```python
from build123d import *

# Parameters (mm, degrees)
EXTRUDE_1_DEPTH     = 50
SKETCH_2_R          = 13
SKETCH_2_R_2        = 2.1
CUT_EXTRUDE_1_DEPTH = 50
FILLET_1_R          = 2
SKETCH_4_R          = 12.5
SKETCH_4_R_2        = 2.5
CUT_EXTRUDE_2_DEPTH = 50
EXTRUDE_2_DEPTH     = 2
EXTRUDE_START       = -50
EXTRUDE_3_DEPTH     = 2


with BuildPart() as part:
    # 草图1 → 凸台-拉伸1 (new body)
    with BuildSketch(Plane.XY):
        with BuildLine():
            Line((0, 0), (46, 0))
            ThreePointArc((46, 0), (48.828427125, 1.171572875), (50, 4))
            Line((50, 4), (50, 50))
            Line((50, 50), (48, 50))
            Line((48, 50), (48, 4))
            ThreePointArc((48, 4), (47.414213562, 2.585786438), (46, 2))
            Line((46, 2), (0, 2))
            Line((0, 2), (0, 0))
        make_face()
    extrude(amount=EXTRUDE_1_DEPTH)

    # 草图2 → 切除-拉伸1 (cut)
    with BuildSketch(Plane(origin=(50, 0, 0), x_dir=(0, 0, -1), z_dir=(1, 0, 0))):
        with Locations((-25, 28)):
            Circle(SKETCH_2_R)
        with Locations((-25, 45.5)):
            Circle(SKETCH_2_R_2)
        with Locations((-7.5, 28)):
            Circle(SKETCH_2_R_2)
        with Locations((-25, 10.5)):
            Circle(SKETCH_2_R_2)
        with Locations((-42.5, 28)):
            Circle(SKETCH_2_R_2)
    extrude(amount=-CUT_EXTRUDE_1_DEPTH, mode=Mode.SUBTRACT)

    # 圆角1
    fillet_1_edges = [part.edges().sort_by_distance(p)[0] for p in [
        (0, 1, 0),
        (49, 50, 50),
        (0, 1, 50),
        (49, 50, 0),
    ]]
    fillet(fillet_1_edges, radius=FILLET_1_R)

    # 草图4 → 切除-拉伸2 (cut)
    with BuildSketch(Plane.XZ):
        with Locations((24, 25)):
            Circle(SKETCH_4_R)
        with Locations((39, 10)):
            Circle(SKETCH_4_R_2)
        with Locations((9, 10)):
            Circle(SKETCH_4_R_2)
        with Locations((9, 40)):
            Circle(SKETCH_4_R_2)
        with Locations((39, 40)):
            Circle(SKETCH_4_R_2)
    extrude(amount=-CUT_EXTRUDE_2_DEPTH, mode=Mode.SUBTRACT)

    # 草图5 → 凸台-拉伸2 (add)
    with BuildSketch(Plane(origin=(0, 0, 0), x_dir=(-1, 0, 0), z_dir=(0, 0, -1))):
        Polygon((-48, 26), (-24, 2), (-48.828427125, 1.171572875), align=None)
    extrude(amount=-EXTRUDE_2_DEPTH)

    # 草图5<2> → 凸台-拉伸3 (add)
    with BuildSketch(Plane(origin=(0, 0, 0), x_dir=(-1, 0, 0), z_dir=(0, 0, -1)).offset(EXTRUDE_START)):
        Polygon((-48, 26), (-24, 2), (-48.828427125, 1.171572875), align=None)
    extrude(amount=EXTRUDE_3_DEPTH)


solid = part.part
```
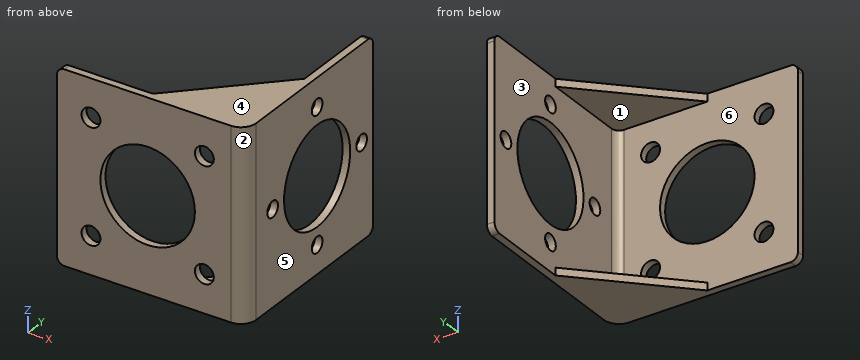
Could you check a few things on this model? Use its own coordinates, in mm. Face numbers are marked on the shaded views. A direction names the side the tool comes from. Coordinates: 2 decimals unless noted, no trailing zeros. Write each loop counter-clockwise with the first axis right and the second up, starting at its lowest first coordinate (ties: lowest second). Pieces come first, ordered by that corner, then holes. Notation, with made-up numbers: (-3, -18.5) -> (52, -18.5) arc R34 cw to (52, 14.5) -> close; hole circle Ø4 at (39, 60.25). An arc over 180 degrees is marked (long way). Return JSON: item names as keys, results as strings.
(1) I'm going to push flat-ended pins straight in: pin 1 (19 mm diameter, centred on x = 39, y = 14, fed in from -Z); pin 2 (23 mm diameter, centred on y = 22.5, z = 29, fed in from -X); pin 3 (12 mm diameter, centred on y = 10.5, z = 5, fed in from -X); pin 4 (14 mm diameter, centred on x = 32, z = 33.5, fed in from +Y). Where does each tip first touch, or does it pass through?
Numbers:
{"pin 1": "stops at z = 0", "pin 2": "stops at x = 48", "pin 3": "stops at x = 27.3", "pin 4": "stops at y = 2"}
(2) Which directions (+Z, -Z, +X, -X, +Y, -Y) give clear straight access to the entire face, cutting with the end or side of a thin tool? Please do the marked faces 1 and 2.
Numbers:
{"face 1": "-X, +Y", "face 2": "+Z, -Z, +X, -Y"}
(3) Imagine slicing it at B-B, the plane x = 44. Please give me the cut outline in (y, z).
Numbers:
{"outline": "(0, 0) -> (22, 0) -> (22, 2) -> (2, 2) -> (2, 48) -> (22, 48) -> (22, 50) -> (0, 50) -> close"}
(4) We'd pull the mould along Z, two halves only. Please class the marked faces 3, 4, 5 and 6: +Z half, -Z half, draft (parallel to the pull), parting line (faces both ways), or undercut.
Numbers:
{"face 3": "undercut", "face 4": "+Z half", "face 5": "draft", "face 6": "undercut"}
(5) Imagine slicing it at C-C, the plane y = 39. Please give me the cut outline in (x, z).
Numbers:
{"outline": "(48, 0) -> (50, 0) -> (50, 18.07) -> (48, 18.07) -> close; (48, 31.93) -> (50, 31.93) -> (50, 50) -> (48, 50) -> close"}
(6) I need wall thicknesses on L1, parallel to Z at x = 9, y = 1; L2, parallel to Z at x = 43, y = 3.5; L3, parallel to Y at x = 49.25, z = 25. Which ranges of each line are inside material? Lowest first, please.
Numbers:
{"L1": "z = 0 to 7.5, 12.5 to 37.5, 42.5 to 50", "L2": "z = 0 to 2, 48 to 50", "L3": "y = 1.67 to 8.4, 12.6 to 15, 41 to 43.4, 47.6 to 50"}
(7) Imagine slicing it at A-A, the plane z = 19. Please give me the cut outline in (x, y), then the cut area to 3 significant figures.
Numbers:
{"outline": "(0, 0) -> (13.03, 0) -> (13.03, 2) -> (0, 2) -> close; (34.97, 0) -> (46, 0) arc R4 ccw to (50, 4) -> (50, 16.47) -> (48, 16.47) -> (48, 4) arc R2 cw to (46, 2) -> (34.97, 2) -> close; (48, 39.53) -> (50, 39.53) -> (50, 50) -> (48, 50) -> close", "area": "103 mm2"}
(8) Imagine slicing it at D-D, the plane y = 6. Please give me the cut outline in (x, z).
Numbers:
{"outline": "(28, 0) -> (50, 0) -> (50, 50) -> (28, 50) -> (28, 48) -> (48, 48) -> (48, 2) -> (28, 2) -> close"}
